CAD build for the part. Positions are in the model's coordinates, mm. A direction names the side the tool comes from. Round coordinates to 2 decimals unless told otherwise and drop trailing zeros. Order: outer loops, then holes, each group sorted by start corner. A loop starts at its lowest first (then second) coordinate and runs counter-clockwise, first axis right, second up. Notation, with made-up numbers: (0.25, 82.5) -> (23.25, 82.5) arc R32 ccw to (23.25, 117.5) -> close; hole circle Ø7 at (-34, 28.25). An arc over 180 degrees is marked (long way). Answer as CSV lines item,"result". Start each with the question number.
from build123d import *

# Parameters (mm, degrees)
BOSS_EXTRUDE1_DEPTH          = 550
CHAMFER6_SIZE                = 31.75
CHAMFER7_SIZE                = 31.75
TOPHOLES_SKETCH3_R           = 1.5875
TOPHOLES_CUT_EXTRUDE2_DEPTH  = 552.656227306
SIDEHOLES_SKETCH4_R          = 1.5875
SIDEHOLES_CUT_EXTRUDE3_DEPTH = 552.656227306


with BuildPart() as part:
    # Sketch1 → Boss-Extrude1 (new body)
    with BuildSketch(Plane(origin=(0, 0, 0), x_dir=(0, 0, -1), z_dir=(1, 0, 0))):
        Polygon((0, 0), (-31.75, 0), (-31.75, 3.175), (-3.175, 3.175), (-3.175, 31.75), (0, 31.75), align=None)
    extrude(amount=BOSS_EXTRUDE1_DEPTH)

    # Chamfer6
    chamfer6_edges = [part.edges().sort_by_distance(p)[0] for p in [
        (550, 1.5875, 31.75),
    ]]
    chamfer(chamfer6_edges, length=CHAMFER6_SIZE - 0.0001)  # a hair under: the kernel refuses the full size

    # Chamfer7
    chamfer7_edges = [part.edges().sort_by_distance(p)[0] for p in [
        (0, 1.5875, 31.75),
    ]]
    chamfer(chamfer7_edges, length=CHAMFER7_SIZE - 0.0001)  # a hair under: the kernel refuses the full size

    # TopHoles-Sketch3 → TopHoles-Cut-Extrude2 (cut, through all)
    with BuildSketch(Plane(origin=(0, 3.175, 0), x_dir=(1, 0, 0), z_dir=(0, 1, 0))):
        with Locations(Location((58.7375, -23.8125, 0), (0, 0, 270))):
            Circle(TOPHOLES_SKETCH3_R)
        with Locations(Location((491.2625, -23.8125, 0), (0, 0, 270))):
            Circle(TOPHOLES_SKETCH3_R)
        with Locations(Location((491.2625, -11.1125, 0), (0, 0, 270))):
            Circle(TOPHOLES_SKETCH3_R)
        with Locations(Location((58.7375, -11.1125, 0), (0, 0, 270))):
            Circle(TOPHOLES_SKETCH3_R)
        with Locations(Location((526.1875, -11.1125, 0), (0, 0, 270))):
            Circle(TOPHOLES_SKETCH3_R)
        with Locations(Location((23.8125, -11.1125, 0), (0, 0, 270))):
            Circle(TOPHOLES_SKETCH3_R)
        with Locations(Location((275, -11.1125, 0), (0, 0, 270))):
            Circle(TOPHOLES_SKETCH3_R)
        with Locations(Location((137.5, -11.1125, 0), (0, 0, 270))):
            Circle(TOPHOLES_SKETCH3_R)
        with Locations(Location((412.5, -11.1125, 0), (0, 0, 270))):
            Circle(TOPHOLES_SKETCH3_R)
    extrude(amount=-TOPHOLES_CUT_EXTRUDE2_DEPTH, mode=Mode.SUBTRACT)

    # SideHoles-Sketch4 → SideHoles-Cut-Extrude3 (cut, through all)
    with BuildSketch(Plane.XY.offset(3.175)):
        with Locations((11.1125, 23.8125)):
            Circle(SIDEHOLES_SKETCH4_R)
        with Locations((529.3625, 23.8125)):
            Circle(SIDEHOLES_SKETCH4_R)
        with Locations((20.6375, 23.8125)):
            Circle(SIDEHOLES_SKETCH4_R)
        with Locations((538.8875, 23.8125)):
            Circle(SIDEHOLES_SKETCH4_R)
        with Locations((11.1125, 11.1125)):
            Circle(SIDEHOLES_SKETCH4_R)
        with Locations((20.6375, 11.1125)):
            Circle(SIDEHOLES_SKETCH4_R)
        with Locations((529.3625, 11.1125)):
            Circle(SIDEHOLES_SKETCH4_R)
        with Locations((538.8875, 11.1125)):
            Circle(SIDEHOLES_SKETCH4_R)
        with Locations((137.5, 11.1125)):
            Circle(SIDEHOLES_SKETCH4_R)
        with Locations((275, 11.1125)):
            Circle(SIDEHOLES_SKETCH4_R)
        with Locations((412.5, 11.1125)):
            Circle(SIDEHOLES_SKETCH4_R)
    extrude(amount=-SIDEHOLES_CUT_EXTRUDE3_DEPTH, mode=Mode.SUBTRACT)


solid = part.part
Item 1: Tool access for faces 1 (the flat face through (271, 16, 0)), 2 (the flat face through (271, 17, 3.175)): list every direction of +Z, -Z, +X, -X, +Y, -Y with a clear straight run to the whole face (end or side of a thin tool).
Item 2: Band-saw the part on A-A, the plane x = 369.5. Give the cut face in (y, z) (3 decimals), and give its area (3 significant figures).
Item 3: Probe line 1 (Y direction, x = 245, z = 21.5) (3 decimals); line 2 (X direction, y = 24, z = 3). List the from-to ranges inside material, lowest first.
Item 4: Pin check, flat tips, straight feed: pin 1 (8 mm diameter, centred on x = 308, y = 16, fed in from +Z) (3 decimals); pin 2 (3.5 mm diameter, centred on x = 491.26, z = 23.81, fed in from +Y) (3 decimals). Stop position of each tip, or through.
Values:
1,face 1,"-Z, +X, -X, +Y, -Y"
1,face 2,"+Z, +X, -X, +Y"
2,outline,"(0, 0) -> (31.75, 0) -> (31.75, 3.175) -> (3.175, 3.175) -> (3.175, 31.75) -> (0, 31.75) -> close"
2,area,"192 mm²"
3,line 1,"0 to 3.175"
3,line 2,"3 to 9.54, 12.69 to 19.06, 22.21 to 527.79, 530.94 to 537.31, 540.46 to 547"
4,pin 1,"z = 3.175"
4,pin 2,"y = 3.175"
